Geometry: see drawing. Coordinates: mm, zero at the bounding-box minimum. A direction names the side the tool comes from. Give positions to 0.01 mm unless a question says otherwise; leave off trailing zeros. Order: outer loops, then holes, each group sorted by start corner. A loop starts at its lowest first (then second) coordinate and runs counter-clockwise, first axis right, second up. Notation, with made-up numbers: (43.25, 0.5) -> (49.25, 0.5) arc R20 cw to (49.25, 29.5) -> close; hole circle Ø10 at (32, -26). An arc over 180 degrees is marked (long way). One line per item, written item: value. Start each with the question number.
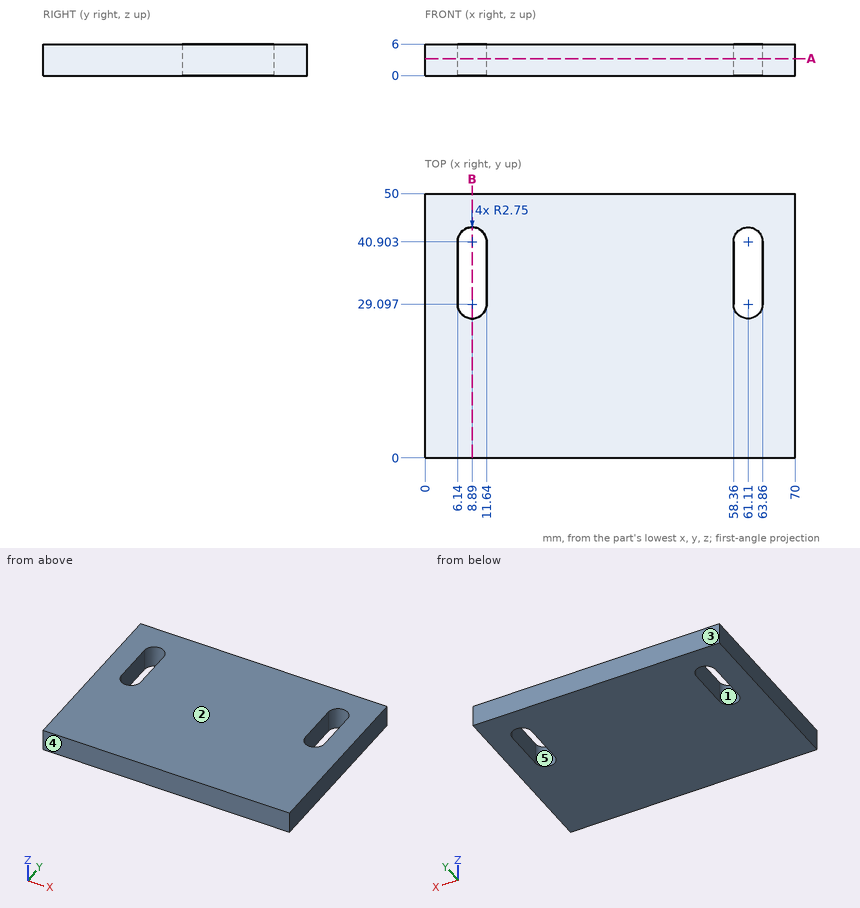
1. Pin query (flat end, axial travel): P1, Ø2, axis at y = 11.5, z = 1, coming from the -X side. Return the tip coordinate at first contact, or that it passes through.
2. Draft query along Y for the marked faces 3, 4 and 5. Return one class per face: pulls with the +Y half, pulls with the -Y half, needs draft (parallel to the pull), parting line crosses it, or undercut.
3. Material intervals for L1, parallel to X at y = 41, z = 0.5; L2, parallel to X at y = 41.5, z = 5.6 (1 decimal); L3, parallel to Y at x = 10, z = 2.35, sorted ascending. Write a range as [from, to].
4. Access query for the marked faces 1 and 2. Directions: +Z, -Z, +X, -X, +Y, -Y. A direction counts if a zero-diameter tool reaches every point of the face in a straight line with its end or side. Return the directions, or none.
5. Cut plane B-B, the plane x = 8.89. Return loops of the section in (y, z).
6. Cut plane A-A, the plane z = 3.25. Return loops of the section in (x, y).
Answers follow:
1. P1: stops at x = 0
2. face 3: pulls with the +Y half
2. face 4: pulls with the -Y half
2. face 5: undercut
3. L1: x = [0, 6.14], [11.64, 58.36], [63.86, 70]
3. L2: x = [0, 6.2], [11.6, 58.4], [63.8, 70]
3. L3: y = [0, 26.58], [43.42, 50]
4. face 1: +Z, -Z
4. face 2: +Z, +X, -X, +Y, -Y
5. outline: (0, 0) -> (26.35, 0) -> (26.35, 6) -> (0, 6) -> close; (43.65, 0) -> (50, 0) -> (50, 6) -> (43.65, 6) -> close
6. outline: (0, 0) -> (70, 0) -> (70, 50) -> (0, 50) -> close; hole (6.14, 29.1) arc R2.75 ccw to (11.64, 29.1) -> (11.64, 40.9) arc R2.75 ccw to (6.14, 40.9) -> close; hole (58.36, 29.1) arc R2.75 ccw to (63.86, 29.1) -> (63.86, 40.9) arc R2.75 ccw to (58.36, 40.9) -> close
